from build123d import *

# Parameters (mm, degrees)
POCKET_DEPTH = 2.3


with BuildPart() as part:
    # Sketch → Revolution (revolve)
    with BuildSketch(Plane.YZ):
        Polygon((0, 0), (0, 5), (0.3, 5), (2.8, 2.5), (9.717098, 2.5), (10, 2.01), (10, 0), align=None)
    revolve(axis=Axis((0, 0, 0), (0, 1, 0)))

    # Sketch001 → Pocket (cut)
    with BuildSketch(Plane(origin=(0, 0, 0), x_dir=(0, 0, -1), z_dir=(0, -1, 0))):
        Polygon((0.866025, 1.5), (-0.866025, 1.5), (-1.732051, 0), (-0.866025, -1.5), (0.866025, -1.5), (1.732051, 0), align=None)
    extrude(amount=-POCKET_DEPTH, mode=Mode.SUBTRACT)


solid = part.part
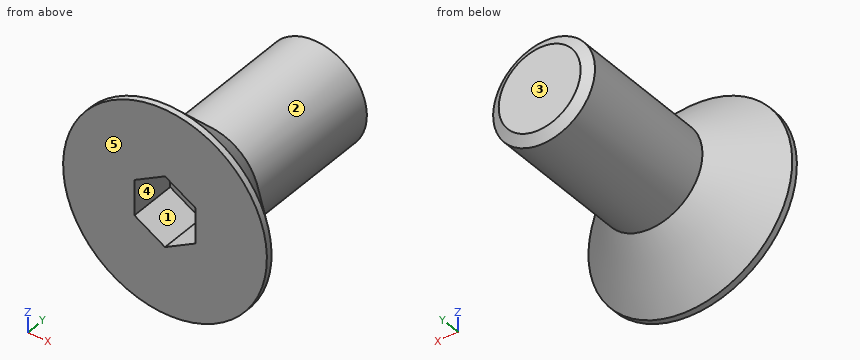
Build history of the part. All positions in model axes, mm. Face numbers are marked on the shaded views. A direction names the side the tool comes from. Round coordinates to 2 decimals unless told otherwise and drop trailing zeros. Loops run counter-clockwise (first coordinate to the right, second up) from the corner with the lowest first, then second, coordinate; pieces in that order, holes last. Notation, with made-up numbers: (43.25, 77.25) -> (95.25, 77.25) arc R14 ccw to (95.25, 88.25) -> close; hole circle Ø6 at (38, 87.25). An arc over 180 degrees is marked (long way). Use CSV: the item, a comma, the result in double quotes. Start each with the question number.
Q1. Saw through at A-A on z = 0. Give the cut face in (x, y).
Q2. Mould opens along X. For the marked faces 1, 2 and 3 say: +X half, -X half, draft (parallel to the pull), parting line (faces both ways), or undercut.
Q3. Which spindle directions (+Z, -Z, +X, -X, +Y, -Y) get a long thin tool onto all of the face, cutting with end or side? Do the marked faces 4 and 5. Say none if no direction does.
Q4. Flat gauge pins, fed straight in: pin 1 Ø3 at (y, z) = (7, 3.5) entering from +X; pin 2 Ø0.9 at (x, z) = (0, 0.5) entering from -Y; pin 3 Ø4 at (x, y) = (3.5, 8) entering from +Z. Where does each tip first touch, or does it go through?
Q5. Saw through at B-B on y = 7. Give the cut face in (x, z), and give its area (3 significant figures).
Q6. Drill centre lines: L1, parallel to Z at x = 2, y = 6.5; L2, parallel to Z at x = -1.25, y = 1.75; L3, parallel to Y at x = 1.25, z = 0. Where is each one in solid material? Low to high.
Solutions:
1,outline,"(-5, 0) -> (-1.5, 0) -> (-1.5, 2.3) -> (1.5, 2.3) -> (1.5, 0) -> (5, 0) -> (5, 0.3) -> (2.5, 2.8) -> (2.5, 9.72) -> (2.01, 10) -> (-2.01, 10) -> (-2.5, 9.72) -> (-2.5, 2.8) -> (-5, 0.3) -> close"
2,face 1,"undercut"
2,face 2,"parting line"
2,face 3,"draft"
3,face 4,"-Y"
3,face 5,"+Z, -Z, +X, -X, -Y"
4,pin 1,"stops at x = 1.5"
4,pin 2,"stops at y = 2.3"
4,pin 3,"stops at z = 2"
5,outline,"circle Ø5 at (0, 0)"
5,area,"19.6 mm^2"
6,L1,"z = -1.5 to 1.5"
6,L2,"z = -3.32 to -1.01, 1.01 to 3.32"
6,L3,"y = 2.3 to 10"
